```python
from build123d import *

# Parameters (mm, degrees)
F0_W           = 12
F0_H           = 25
F1_DEPTH       = 10
F2_R           = 10
F3_DEPTH       = 23
F5_DEPTH       = 25
F7_D           = 4.4
F7_CSINK_D     = 8.96
F7_CSINK_ANGLE = 90


with BuildPart() as f1:
    # F0 (on Front) → F1 (new body)
    with BuildSketch(Plane.XZ):
        with Locations((6, 12.5)):
            Rectangle(F0_W, F0_H)
    extrude(amount=F1_DEPTH)

    # F2 (on face) → F3 (cut)
    with BuildSketch(Plane(origin=(0, 0, 0), x_dir=(1, 0, 0), z_dir=(0, 0, -1))):
        with Locations((6, -4)):
            Circle(F2_R)
    extrude(amount=-F3_DEPTH, mode=Mode.SUBTRACT)

    # F4 (on face) → F5 (cut)
    with BuildSketch(Plane.XY.offset(25)):
        with BuildLine():
            ThreePointArc((6, -4), (8.8284271247, -2.8284271247), (10, 0))
            ThreePointArc((10, 0), (3.1715728753, 2.8284271247), (6, -4))
        make_face()
        with BuildLine():
            Line((0, -4), (6, -4))
            ThreePointArc((6, -4), (3.1715728753, -2.8284271247), (2, 0))
            Line((2, 0), (0, 0))
            Line((0, 0), (0, -4))
        make_face()
    extrude(amount=-F5_DEPTH, mode=Mode.SUBTRACT)

    # F7 (through all)
    with Locations(Plane.XZ.offset(10)):
        with Locations((6, 6), (6, 16)):
            CounterSinkHole(F7_D / 2, F7_CSINK_D / 2, counter_sink_angle=F7_CSINK_ANGLE)


solid = f1.part
```
Read the model definition and answer for the solid it produces. Units are mm, in the model's axes. A direction names the side the tool comes from. Give positions to 0.01 mm unless a question says otherwise; leave off trailing zeros. Loops run counter-clockwise (first coordinate to the right, second up) from the corner with the lowest first, then second, coordinate; pieces in that order, holes last.
Item 1: The part is cut by section A-A (z = 16). Write down the section's boundary in (x, y) (3 decimals), and give its area (3 significant figures).
Item 2: Find the intervals of material crossed by line 1 along Z through (x, y) = (6, -7); line 2 along X through (y, z) = (-6.75, 6); line 3 along Z through (x, y) = (7.75, -6.25), in increasing order.
Item 3: The mould has two halves that part along Z. Classify faces 3 (the conical face through (6.3, -7.83, 8.29)), 4 (the flat face through (3, -4, 24)), 5 (the flat face through (7, -6, 25)), 6 (the flat face through (7.2, -4.4, 23)): released by +Z, released by -Z, zero draft, split by the parting line, or undercut.
Item 4: The part is cut by section B-B (y = -6.25). Write down the section's boundary in (x, z).
Item 5: Each of these flat-tipped pins is pushed along its axis until it touches: pin 1 Ø6 at (x, y) = (9.5, -2) entering from -Z; pin 2 Ø1 at (x, z) = (3, 23.5) entering from +Y. Where does it stop, or does it pass through?
Item 6: For faces 1 (the cylindrical face through (6, -6, 11)), 2 (the cylindrical face through (3.9, -6.72, 6.66)), determine the directions among +Z, -Z, +X, -X, +Y, -Y from which every point of the face is accessible in a straight line to the end or side of a thin tool.
Item 7: The part is cut by section C-C (x = 5.75). Give the number of separate pieces and of enclosed holes in the cut face, and give its area (3 significant figures).
Item 8: The part is cut by section D-D (z = 21.25). Write down the section's boundary in (x, y), and give its area (4 significant figures).
Taken from the geometry:
1. outline: (0, -10) - (1.52, -10) - (3.8, -7.72) - (3.8, -5.755) arc R10 cw to (0, -4) - close; (8.2, -7.72) - (10.48, -10) - (12, -10) - (12, -4) arc R10 cw to (8.2, -5.755) - close
1. area: 32.5 mm2
2. line 1: z = 0 to 3.8, 8.2 to 13.8, 18.2 to 25
2. line 2: x = 0 to 3.8, 8.2 to 12
2. line 3: z = 0 to 4.67, 7.33 to 14.67, 17.33 to 25
3. face 3: undercut
3. face 4: zero draft
3. face 5: released by +Z
3. face 6: released by -Z
4. outline: (0, 0) - (12, 0) - (12, 25) - (0, 25) - close; hole circle Ø4.4 at (6, 6); hole circle Ø4.4 at (6, 16)
5. pin 1: stops at z = 23
5. pin 2: stops at y = -4
6. face 1: -Z, +Y
6. face 2: +Y, -Y
7. separate pieces: 3
7. enclosed holes: 0
7. area: 58.6 mm2
8. outline: (0, -10) - (12, -10) - (12, -4) arc R10 cw to (0, -4) - close
8. area: 55.65 mm2
